```python
from build123d import *

# Parameters (mm, degrees)
F0_R     = 10
F1_DEPTH = 5


with BuildPart() as f1:
    # F0 (on Top) → F1 (new body)
    with BuildSketch(Plane.XY):
        with BuildLine():
            ThreePointArc((-79.890026, 0), (-79.182919, 0.292893), (-78.890026, 1))
            Line((-78.890026, 1), (-78.890026, 44.5))
            ThreePointArc((-78.890026, 44.5), (-78.597133, 45.207107), (-77.890026, 45.5))
            Line((-77.890026, 45.5), (-70.890026, 45.5))
            ThreePointArc((-70.890026, 45.5), (-70.182919, 45.207107), (-69.890026, 44.5))
            Line((-69.890026, 44.5), (-69.890026, 0))
            Line((-69.890026, 0), (66.528554, 56.729136))
            ThreePointArc((66.528554, 56.729136), (70.581868, 60.793756), (70.573874, 66.534002))
            Line((70.573874, 66.534002), (62.493371, 85.965476))
            ThreePointArc((62.493371, 85.965476), (58.938302, 89.785922), (53.751584, 90.362352))
            Line((53.751584, 90.362352), (-82.20672, 56.418899))
            ThreePointArc((-82.20672, 56.418899), (-86.30083, 53.758785), (-87.890026, 49.142249))
            Line((-87.890026, 49.142249), (-87.890026, 1))
            ThreePointArc((-87.890026, 1), (-87.597133, 0.292893), (-86.890026, 0))
            Line((-86.890026, 0), (-79.890026, 0))
        make_face()
        Polygon((-62.390026, 53.636143), (-10.687523, 66.544229), (-39.176145, 20.894883), (-62.390026, 11.241481), align=None, mode=Mode.SUBTRACT)
        Polygon((-30.880324, 24.344668), (-3.410874, 68.360923), (24.289399, 75.359991), (0.629378, 37.447855), align=None, mode=Mode.SUBTRACT)
        Polygon((9.017346, 40.935959), (31.585224, 77.098076), (40.997005, 54.46523), align=None, mode=Mode.SUBTRACT)
        with Locations((50.109974, 70.167761)):
            Circle(F0_R, mode=Mode.SUBTRACT)
    extrude(amount=F1_DEPTH)


solid = f1.part
```
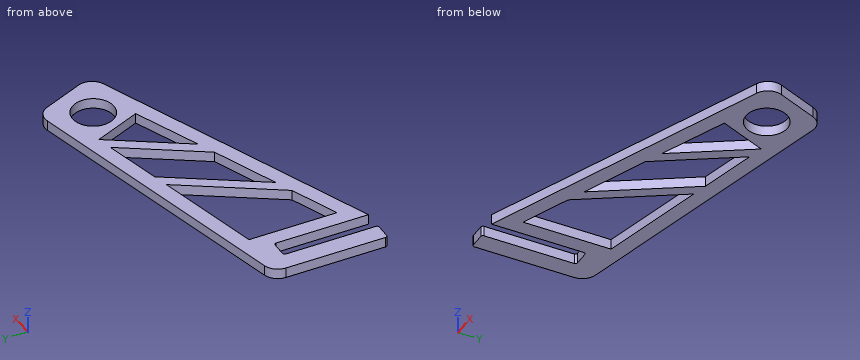
Model file for the job. Use its own axes, mm. Give positions to 0.01 mm unless a question says otherwise; leave off trailing zeros. Write each loop counter-clockwise with the first axis right and the second up, starting at its lowest first coordinate (ties: lowest second). Pieces come first, ordered by that corner, then holes. Notation, with made-up numbers: (53.25, -21.75) -> (83.25, -21.75) arc R35 ccw to (83.25, 17.25) -> close; hole circle Ø9 at (44.5, 45.5). An arc over 180 degrees is marked (long way). Use CSV: the item, a comma, the result in double quotes. Start each with the question number.
1) Cut at D-D on x = 3. List the corners of the cut face in (y, z), plus the area to 3 significant figures.
2) Cut at A-A on x = 44. List the corners of the cut face in (y, z).
3) Pin check, flat tips, straight feed: P1, Ø1.5, axis at x = 2, z = 3.5, coming from the +Y side; P2, Ø18, axis at x = 50.11, y = 70.17, coming from the +Z side; P3, Ø1.5, axis at y = 23.5, z = 3, coming from the +X side; P4, Ø1.5, axis at x = -13, z = 1.5, coming from the +Y side. Stop position of each tip, or through.
4) Drill centre lines: L1, parallel to X at y = 48, z = 1.8; L2, parallel to Y at x = -17.5, z = 1.65; L3, parallel to X at y = 34.5, z = 1.45. Where is each one in solid material? Low to high.
5) Cut at C-C on z = 1.25. List the corners of the cut face in (x, y), plus the area to 3 significant figures.
6) Cut at B-B on y = 28. List the corners of the cut face in (x, z), plus the area to 3 significant figures.
Final values:
1,outline,"(30.31, 0) -> (41.25, 0) -> (41.25, 5) -> (30.31, 5) -> close; (69.98, 0) -> (77.69, 0) -> (77.69, 5) -> (69.98, 5) -> close"
1,area,"93.2 mm2"
2,outline,"(47.36, 0) -> (62.25, 0) -> (62.25, 5) -> (47.36, 5) -> close; (78.08, 0) -> (87.93, 0) -> (87.93, 5) -> (78.08, 5) -> close"
3,P1,"stops at y = 77.63"
3,P2,"passes through"
3,P3,"stops at x = -11.58"
3,P4,"stops at y = 73.88"
4,L1,"x = -87.89 to -62.39, -22.26 to -16.12, 7.21 to 13.43, 25.71 to 45.54"
4,L2,"y = 21.79 to 29.91, 45.78 to 55.63, 64.84 to 72.57"
4,L3,"x = -87.89 to -78.89, -69.89 to -62.39, -30.69 to -24.54, -6.46 to 13.07"
5,outline,"(-87.89, 1) arc R1 ccw to (-86.89, 0) -> (-79.89, 0) arc R1 ccw to (-78.89, 1) -> (-78.89, 44.5) arc R1 cw to (-77.89, 45.5) -> (-70.89, 45.5) arc R1 cw to (-69.89, 44.5) -> (-69.89, 0) -> (66.53, 56.73) arc R7.5 ccw to (70.57, 66.53) -> (62.49, 85.97) arc R7.5 ccw to (53.75, 90.36) -> (-82.21, 56.42) arc R7.5 ccw to (-87.89, 49.14) -> close; hole (-62.39, 11.24) -> (-39.18, 20.89) -> (-10.69, 66.54) -> (-62.39, 53.64) -> close; hole (-30.88, 24.34) -> (0.63, 37.45) -> (24.29, 75.36) -> (-3.41, 68.36) -> close; hole (9.02, 40.94) -> (41, 54.47) -> (31.59, 77.1) -> close; hole circle Ø20 at (50.11, 70.17)"
5,area,"3,990 mm2"
6,outline,"(-87.89, 0) -> (-78.89, 0) -> (-78.89, 5) -> (-87.89, 5) -> close; (-69.89, 0) -> (-62.39, 0) -> (-62.39, 5) -> (-69.89, 5) -> close; (-34.74, 0) -> (-28.6, 0) -> (-28.6, 5) -> (-34.74, 5) -> close; (-22.09, 0) -> (-2.56, 0) -> (-2.56, 5) -> (-22.09, 5) -> close"
6,area,"211 mm2"
